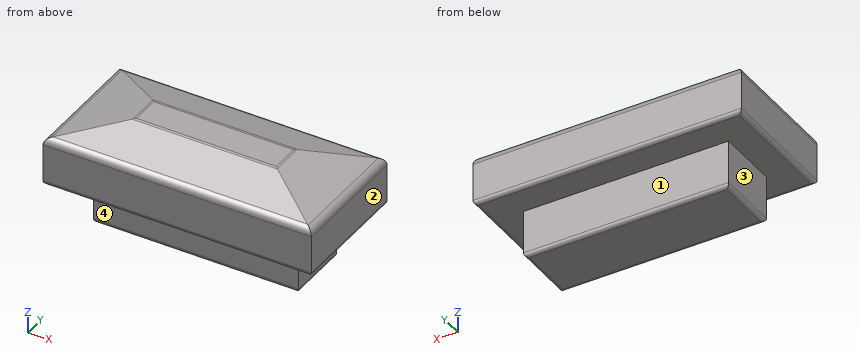
Solid Edge part; units mm, degrees
sketch "Sketch1" plane through (0, 0, 0) normal (0, 0, 1) x (1, 0, 0)
  line L0 (-8.5, -4) -> (8.5, -4)
  line L1 (8.5, -4) -> (8.5, 4)
  line L2 (8.5, 4) -> (-8.5, 4)
  line L3 (-8.5, 4) -> (-8.5, -4)
  dimension "D1" = 8.5
  dimension "D2" = 8.5
extrude "Protrusion1" add sketch "Sketch1" against normal blind 6
sketch "Sketch2" plane through (0, 0, -6) normal (0, 0, -1) x (1, 0, 0)
  line L0 (-6.5, -2) -> (6.5, -2)
  line L1 (6.5, -2) -> (6.5, 2)
  line L2 (6.5, 2) -> (-6.5, 2)
  line L3 (-6.5, 2) -> (-6.5, -2)
  dimension "D1" = 6.5
  dimension "D2" = 6.5
extrude "Extrusionsausschnitt_1" cut sketch "Sketch2" against normal blind 3 flip side to cut
fillet "Verrundung_1" radius 0.25 8 edges at (0, -2, -6) (6.5, 0, -6) (0, 2, -6) (-6.5, 0, -6) (0, -4, -3) (8.5, 0, -3) (0, 4, -3) (-8.5, 0, -3)
sketch "Sketch3" plane through (0, 0, 0) normal (0, 0, 1) x (1, 0, 0)
  line L0 (-4.5, -1) -> (4.5, -1)
  line L1 (4.5, -1) -> (4.5, 1)
  line L2 (4.5, 1) -> (-4.5, 1)
  line L3 (-4.5, 1) -> (-4.5, -1)
  dimension "D1" = 4.5
  dimension "D2" = 4.5
extrude "Extrusionsausprägung_2" add sketch "Sketch3" along normal blind 1
sketch "Sketch4" plane through (4.5, 0, 0.5) normal (1, 0, 0) x (0, 1, 0)
  line L0 (-4, -0.5) -> (-1, 0.5)
  line L1 (-4, -0.5) -> (4, -0.5)
  line L2 (1, 0.5) -> (4, -0.5)
  line L3 (-1, 0.5) -> (1, 0.5)
extrude "Extrusionsausprägung_3" add sketch "Sketch4" against normal blind 13 and the other way blind 4
sketch "Sketch5" plane through (0, -4, -1.375) normal (0, -1, 0) x (1, 0, 0)
  line L0 (-8.5, 1.375) -> (-4.5, 2.375)
  line L1 (-4.5, 2.375) -> (4.5, 2.375)
  line L2 (4.5, 2.375) -> (8.5, 1.375)
  dimension "D1" = 4.5
extrude "Extrusionsausschnitt_2" cut sketch "Sketch5" against normal blind 10 material side at (-6.5121, -4, 0.5485)
fillet "Verrundung_4" radius 0.5 8 edges at (0, -1, 1) (-4.5, 0, 1) (0, 1, 1) (4.5, 0, 1) (0, -4, 0) (8.5, 0, 0) (0, 4, 0) (-8.5, 0, 0)
properties part number "053" material "PLA"
Geometry: final body of the model. Coordinates: model frame, mm. Face numbers are marked on the shaded views. A direction names the side the tool comes from. Round coordinates to 2 decimals unless told otherwise and drop trailing zeros. Loops run counter-clockwise (first coordinate to the right, second up) from the corner with the lowest first, then second, coordinate; pieces in that order, holes last.
Q1. Section C-C on z = -5.25. Return loops of the section in (x, y).
Q2. Section A-A on y = -0.5. Return loops of the section in (x, z).
Q3. Access query for the marked faces 1, 2, 3 and 4. Directions: +Z, -Z, +X, -X, +Y, -Y. A direction counts if a zero-diameter tool reaches every point of the face in a straight line with its end or side. Return the directions, or none.
Q4. Section D-D on y = 2.25. Return loops of the section in (x, z), plus the area to 3 significant figures.
Q5. Pin query (flat end, axial travel): P1, Ø2, axis at y = 0.5, z = -5, coming from the +X side; P2, Ø2, axis at x = -2, z = -4.5, coming from the -Y side; P3, Ø1.4, axis at y = 0.5, z = -4, coming from the -X side. Return the tip coordinate at first contact, or that it passes through.
Q6. Section B-B on x = 0.75. Return loops of the section in (y, z).
Q7. Material intervals for L1, parallel to Y at x = -3.25, z = -4.75; L2, parallel to Z at x = 3.75, y = -1.25; L3, parallel to X at y = 0, z = -4.75, sorted ascending.
Evaluation:
1. outline: (-6.5, -2) - (6.5, -2) - (6.5, 2) - (-6.5, 2) - close
2. outline: (-8.5, -2.75) arc R0.25 ccw to (-8.25, -3) - (-6.5, -3) - (-6.5, -5.75) arc R0.25 ccw to (-6.25, -6) - (6.25, -6) arc R0.25 ccw to (6.5, -5.75) - (6.5, -3) - (8.25, -3) arc R0.25 ccw to (8.5, -2.75) - (8.5, -0.39) arc R0.5 ccw to (8.12, 0.09) - (4.56, 0.99) arc R0.5 ccw to (4.44, 1) - (-4.44, 1) arc R0.5 ccw to (-4.56, 0.99) - (-8.12, 0.09) arc R0.5 ccw to (-8.5, -0.39) - close
3. face 1: -Z, +X, -X, +Y
3. face 2: +Z, -Z, +X, +Y, -Y
3. face 3: -Z, -X, +Y, -Y
3. face 4: -Z, +X, -X, -Y
4. outline: (-8.5, -2.75) arc R0.25 ccw to (-8.25, -3) - (8.25, -3) arc R0.25 ccw to (8.5, -2.75) - (8.5, -0.39) arc R0.5 ccw to (8.12, 0.09) - (6.17, 0.58) - (-6.17, 0.58) - (-8.12, 0.09) arc R0.5 ccw to (-8.5, -0.39) - close
4. area: 59.5 mm2
5. P1: stops at x = 6.5
5. P2: stops at y = -2
5. P3: stops at x = -6.5
6. outline: (-4, -2.75) arc R0.25 ccw to (-3.75, -3) - (-2, -3) - (-2, -5.75) arc R0.25 ccw to (-1.75, -6) - (1.75, -6) arc R0.25 ccw to (2, -5.75) - (2, -3) - (3.75, -3) arc R0.25 ccw to (4, -2.75) - (4, -0.36) arc R0.5 ccw to (3.66, 0.11) - (1.08, 0.97) arc R0.5 ccw to (0.92, 1) - (-0.92, 1) arc R0.5 ccw to (-1.08, 0.97) - (-3.66, 0.11) arc R0.5 ccw to (-4, -0.36) - close
7. L1: y = -2 to 2
7. L2: z = -6 to 0.92
7. L3: x = -6.5 to 6.5
